from build123d import *

# Parameters (mm, degrees)
F0_W     = 128.67894
F0_H     = 27.281861
F0_R     = 1.7272
F0_W_2   = 106.45394
F0_H_2   = 11.406861
F1_DEPTH = 1.70942
F2_R     = 1.98374
F3_R     = 0.762


with BuildPart() as f1:
    # F0 (on Top) → F1 (new body)
    with BuildSketch(Plane.XY):
        with Locations((64.33947, -13.64093)):
            Rectangle(F0_W, F0_H)
        with Locations((23.313111, -23.313111)):
            Circle(F0_R, mode=Mode.SUBTRACT)
        with Locations((105.365829, -23.313111)):
            Circle(F0_R, mode=Mode.SUBTRACT)
        with Locations((3.96875, -3.96875)):
            Circle(F0_R, mode=Mode.SUBTRACT)
        with Locations((64.33947, -10.46593)):
            Rectangle(F0_W_2, F0_H_2, mode=Mode.SUBTRACT)
        with Locations((124.71019, -3.96875)):
            Circle(F0_R, mode=Mode.SUBTRACT)
    extrude(amount=F1_DEPTH)

    # F2
    f2_edges = [f1.edges().sort_by_distance(p)[0] for p in [
        (0, -27.281861, 0.85471),
        (128.67894, -27.281861, 0.85471),
    ]]
    fillet(f2_edges, radius=F2_R)

    # F3
    f3_edges = [f1.edges().sort_by_distance(p)[0] for p in [
        (0, 0, 0.85471),
        (128.67894, 0, 0.85471),
    ]]
    fillet(f3_edges, radius=F3_R)


solid = f1.part
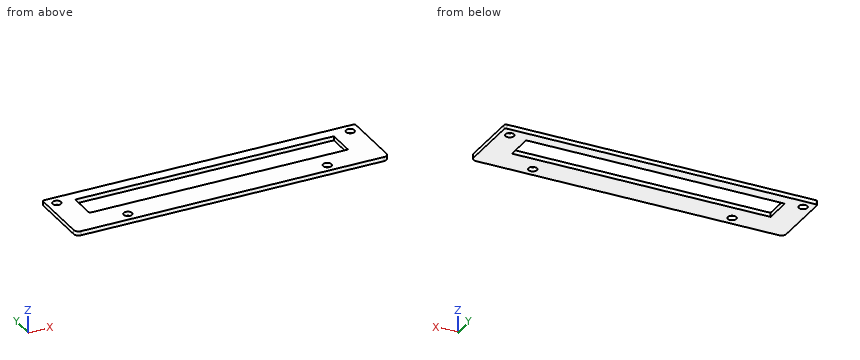
Geometry check sheet. Reference: the model listing, model coordinates, mm. Round coordinates to 2 decimals unless told otherwise and drop trailing zeros. Order: outer loops, then holes, each group sorted by start corner. A loop starts at its lowest first (then second) coordinate and runs counter-clockwise, first axis right, second up. Notation, with made-up numbers: M 22.5,11.5 L 70.5,11.5 A21 ccw 70.5,23.5 Z; hole C 64.25,27 d3. An arc over 180 degrees is marked long. Answer in a Markdown table with one row per item.
(1) Sectioned sample at A-A, the plane y = -10.25. Record the cut outline in (x, z).
Responses:
| item | result |
|---|---|
| outline | M 0,0 L 11.11,0 L 11.11,1.71 L 0,1.71 Z; M 117.57,0 L 128.68,0 L 128.68,1.71 L 117.57,1.71 Z |
(2) Scan lines: probe 1 along Y at (x, z) = (100.5, 1.4); probe 2 along X at (y, z) = (-21.75, 1.15); probe 3 along X at (y, z) = (-12.5, 0.65). Record each from-to range of solid material in increasing order. Write a range as from..to.
Responses:
| item | result |
|---|---|
| probe 1 | y = -27.28..-16.17, -4.76..0 |
| probe 2 | x = 0..22.58, 24.05..104.63, 106.1..128.68 |
| probe 3 | x = 0..11.11, 117.57..128.68 |
(3) Sectioned sample at C-C, the plane z = 1.25. Record the cut outline in (x, y), and give its area (3 significant figures).
Responses:
| item | result |
|---|---|
| outline | M 0,-25.3 A1.98 ccw 1.98,-27.28 L 126.7,-27.28 A1.98 ccw 128.68,-25.3 L 128.68,-0.76 A0.76 ccw 127.92,0 L 0.76,0 A0.76 ccw 0,-0.76 Z; hole C 3.97,-3.97 d3.45; hole M 11.11,-16.17 L 117.57,-16.17 L 117.57,-4.76 L 11.11,-4.76 Z; hole C 23.31,-23.31 d3.45; hole C 105.37,-23.31 d3.45; hole C 124.71,-3.97 d3.45 |
| area | 2,260 mm² |
(4) Sectioned sample at B-B, the plane x = 113. Record the cut outline in (y, z).
Responses:
| item | result |
|---|---|
| outline | M -27.28,0 L -16.17,0 L -16.17,1.71 L -27.28,1.71 Z; M -4.76,0 L 0,0 L 0,1.71 L -4.76,1.71 Z |
